```python
from build123d import *

# Parameters (mm, degrees)
F1_DEPTH = 4
F2_DEPTH = 2


with BuildPart() as f1:
    # F0 (on Front) → F1 (new body)
    with BuildSketch(Plane.XZ):
        with BuildLine():
            ThreePointArc((-36.017278, 29.398246), (-35.326827, 27.208416), (-33.290161, 26.148194))
            Line((-33.290161, 26.148194), (-32.484752, 26.07773))
            ThreePointArc((-32.484752, 26.07773), (-30.253575, 26.803519), (-29.227186, 28.913363))
            Line((-29.227186, 28.913363), (-28.537242, 35.103315))
            Line((-28.537242, 35.103315), (-20.148152, 34.356556))
            Line((-20.148152, 34.356556), (-21.33208, 17.72593))
            Line((-21.33208, 17.72593), (-10.161562, 6.577645))
            ThreePointArc((-10.161562, 6.577645), (-2.155933, 3.368806), (5.701012, 6.926216))
            Line((5.701012, 6.926216), (29.425626, 49.089231))
            ThreePointArc((29.425626, 49.089231), (26.2619, 55.67029), (19.036789, 54.613281))
            Line((19.036789, 54.613281), (-3.875086, 13.894653))
            Line((-3.875086, 13.894653), (-13.112814, 19.599447))
            Line((-13.112814, 19.599447), (-12.160234, 32.994758))
            ThreePointArc((-12.160234, 32.994758), (-13.425174, 36.986259), (-17.083313, 39.023455))
            Line((-17.083313, 39.023455), (-31.851361, 40.322261))
            ThreePointArc((-31.851361, 40.322261), (-34.014612, 39.655086), (-35.095724, 37.666124))
            Line((-35.095724, 37.666124), (-36.017278, 29.398246))
        make_face()
        Polygon((23.022137, 47.828823), (1.829196, 10.165058), (-1.569676, 12.077562), (19.623265, 49.741327), align=None, mode=Mode.SUBTRACT)
    extrude(amount=F1_DEPTH)

    # F0 (on Front) → F2 (join)
    with BuildSketch(Plane.XZ):
        with BuildLine():
            ThreePointArc((-36.017278, 29.398246), (-35.326827, 27.208416), (-33.290161, 26.148194))
            Line((-33.290161, 26.148194), (-32.484752, 26.07773))
            ThreePointArc((-32.484752, 26.07773), (-30.253575, 26.803519), (-29.227186, 28.913363))
            Line((-29.227186, 28.913363), (-28.537242, 35.103315))
            Line((-28.537242, 35.103315), (-20.148152, 34.356556))
            Line((-20.148152, 34.356556), (-21.33208, 17.72593))
            Line((-21.33208, 17.72593), (-10.161562, 6.577645))
            ThreePointArc((-10.161562, 6.577645), (-2.155933, 3.368806), (5.701012, 6.926216))
            Line((5.701012, 6.926216), (29.425626, 49.089231))
            ThreePointArc((29.425626, 49.089231), (26.2619, 55.67029), (19.036789, 54.613281))
            Line((19.036789, 54.613281), (-3.875086, 13.894653))
            Line((-3.875086, 13.894653), (-13.112814, 19.599447))
            Line((-13.112814, 19.599447), (-12.160234, 32.994758))
            ThreePointArc((-12.160234, 32.994758), (-13.425174, 36.986259), (-17.083313, 39.023455))
            Line((-17.083313, 39.023455), (-31.851361, 40.322261))
            ThreePointArc((-31.851361, 40.322261), (-34.014612, 39.655086), (-35.095724, 37.666124))
            Line((-35.095724, 37.666124), (-36.017278, 29.398246))
        make_face()
        Polygon((23.022137, 47.828823), (1.829196, 10.165058), (-1.569676, 12.077562), (19.623265, 49.741327), align=None, mode=Mode.SUBTRACT)
        Polygon((-1.569676, 12.077562), (1.829196, 10.165058), (23.022137, 47.828823), (19.623265, 49.741327), align=None)
    extrude(amount=-F2_DEPTH)


solid = f1.part
```
Verification items for the finished model (mm, model axes). A direction names the side the tool comes from. Coordinates: 2 decimals unless noted, no trailing zeros. Order: outer loops, then holes, each group sorted by start corner. A loop starts at its lowest first (then second) coordinate and runs counter-clockwise, first axis right, second up. Notation, with made-up numbers: (28, 53.25) - (78, 53.25) arc R19 cw to (78, 58.25) - close; hole circle Ø11 at (46.5, -2). An arc over 180 degrees is marked (long way). Return JSON: item names as keys, results as strings.
(1) Section check B-B, the plane z = 27. Record the cut outline in (x, y), and give its area (3 significant figures).
Filled sheet:
{"outline": "(-35.13, -4) - (-30.05, -4) - (-30.05, 2) - (-35.13, 2) - close; (-20.67, -4) - (-12.59, -4) - (-12.59, 2) - (-20.67, 2) - close; (3.5, -4) - (6.83, -4) - (6.83, 0) - (11.3, 0) - (11.3, -4) - (17, -4) - (17, 2) - (3.5, 2) - close", "area": "142 mm^2"}
(2) Section check D-D, the plane x = 10.5. Record the cut outline in (y, z), and give its area (3 significant figures).
Filled sheet:
{"outline": "(-4, 15.45) - (2, 15.45) - (2, 39.44) - (-4, 39.44) - (-4, 33.53) - (0, 33.53) - (0, 25.57) - (-4, 25.57) - close", "area": "112 mm^2"}
(3) Thickness scan on line 1 along X through (y, z) = (-3.3, 26); line 2 along X through (y, z) = (-2.45, 15); line 3 along X through (y, z) = (0.55, 14). Record the ranges inside material, lowest first.
Filled sheet:
{"line 1": "x = -20.74 to -12.66, 2.94 to 6.26, 10.74 to 16.43", "line 2": "x = -18.6 to -5.66, -3.25 to 0.07, 4.55 to 10.24", "line 3": "x = -17.6 to -4.05, -3.82 to 9.68"}
(4) Mould release check, pull along Z, two halves, no side actions. Record for faces 1 (the flat face through (4, 2, 24)), 2 (the flat face through (8.88, -1.97, 30.65)), 3 (the cylindrical face through (-33.989, -1.042, 39.676)): pulls with the +Z half, pulls with the -Z half, needs draft (parallel to the pull), parting line crosses it, or undercut.
Filled sheet:
{"face 1": "needs draft", "face 2": "undercut", "face 3": "pulls with the +Z half"}
(5) Access from +Z, -Z, +X, -X, +Y, -Y to the whole of each face (thin tool, end or side, straight path). Record for faces 4 (the flat face through (-20.73, -1.04, 26.16)), 5 (the flat face through (-24.364, -1.042, 39.664)), 6 (the flat face through (12.574, -1.972, 29.261)).
Filled sheet:
{"face 4": "+Y, -Y", "face 5": "+Z, +Y, -Y", "face 6": "-Y"}
(6) Go/stop test with flat-tipped pins: pin 1 (2 mm diameter, centred on x = -29, y = -3.5, fed in from +Z); pin 2 (12 mm diameter, centred on x = 0, z = 21.5, fed in from -Y); pin 3 (1.5 mm diameter, centred on y = 1, z = 16.5, fed in from +X); pin 4 (1 mm diameter, centred on y = -1, z = 23.5, fed in from +X). Record where each tip stops, or that it passes through.
Filled sheet:
{"pin 1": "stops at z = 40.16", "pin 2": "stops at y = -4", "pin 3": "stops at x = 11.51", "pin 4": "stops at x = 15.31"}
(7) Section check C-C, the plane z = 21.5. Record the cut outline in (x, y).
Filled sheet:
{"outline": "(-21.06, -4) - (-12.98, -4) - (-12.98, 2) - (-21.06, 2) - close; (0.4, -4) - (3.73, -4) - (3.73, 0) - (8.21, 0) - (8.21, -4) - (13.9, -4) - (13.9, 2) - (0.4, 2) - close"}
(8) Section check A-A, the plane y = -1.7. Record the cut outline in (x, z).
Filled sheet:
{"outline": "(-36.02, 29.4) arc R3 ccw to (-33.29, 26.15) - (-32.48, 26.08) arc R3 ccw to (-29.23, 28.91) - (-28.54, 35.1) - (-20.15, 34.36) - (-21.33, 17.73) - (-10.16, 6.58) arc R10.99 ccw to (5.7, 6.93) - (29.43, 49.09) arc R6.16 ccw to (19.04, 54.61) - (-3.88, 13.89) - (-13.11, 19.6) - (-12.16, 32.99) arc R5.67 ccw to (-17.08, 39.02) - (-31.85, 40.32) arc R3 ccw to (-35.1, 37.67) - close; hole (-1.57, 12.08) - (1.83, 10.17) - (23.02, 47.83) - (19.62, 49.74) - close"}
